Input: dimensioned drawing with shaded views. Units: mm. Origin: part minimum x, y, z. A direction names the side the tool comes from. Give positions to 0.01 mm unless a question says otherwise; leave off trailing zeros. Write each loop counter-clockwise with the first axis right and the second up, starting at its lowest first coordinate (ties: lowest second). Pieces come first, ordered by that corner, then holes. Notation, with made-up numbers: M 10.5,44 L 46.5,44 A28 cw 46.5,69 Z; hole C 24,78 d7. An arc over 180 degrees is marked long. Answer as a JSON object with one key per item and string values.
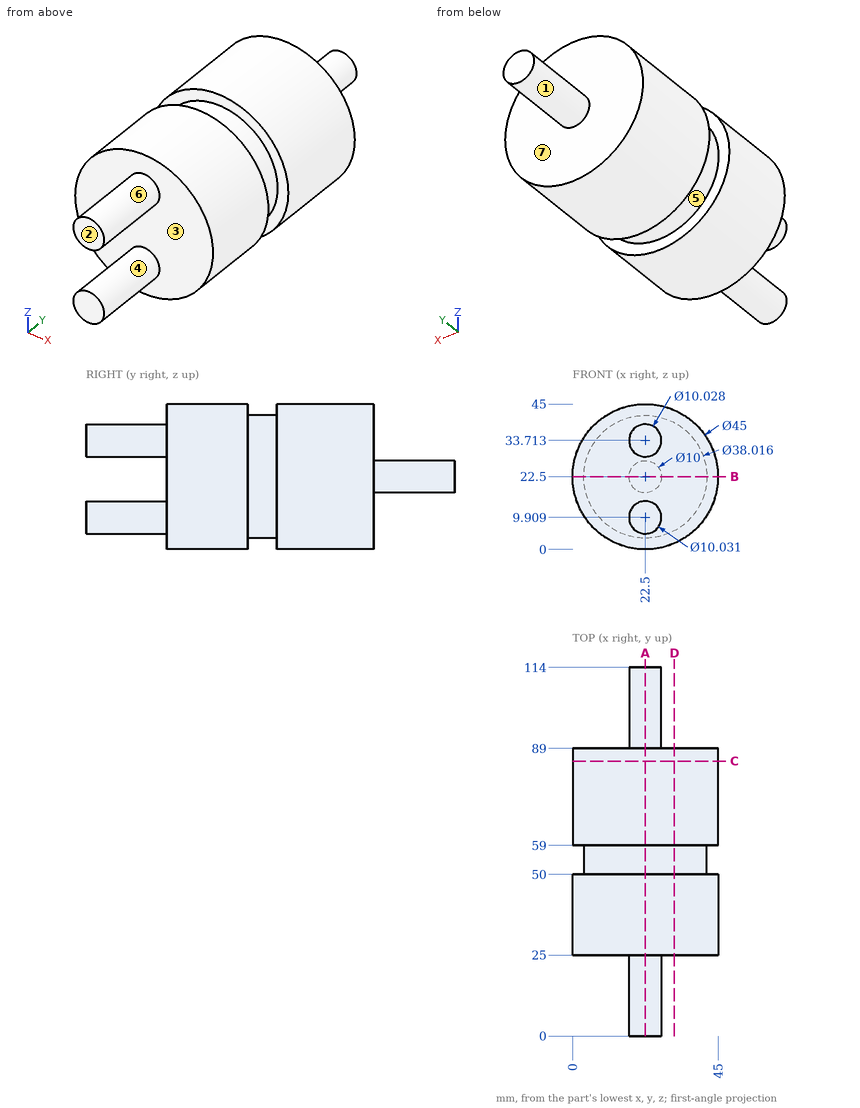
1) Cut plane A-A on x = 22.5. Return loops of the section in (y, z) (1 decimal), and give its area (3 significant figures).
Geometry check:
{"outline": "M 0,4.9 L 25,4.9 L 25,0 L 50,0 L 50,3.5 L 59,3.5 L 59,0 L 89,0 L 89,17.5 L 114,17.5 L 114,27.5 L 89,27.5 L 89,45 L 59,45 L 59,41.5 L 50,41.5 L 50,45 L 25,45 L 25,38.7 L 0,38.7 L 0,28.7 L 25,28.7 L 25,14.9 L 0,14.9 Z", "area": "3,570 mm2"}
2) Contact query for flat-ended pins moving along their axis: P1, Ø3, axis at x = 24.5, y = 67, coming from the +Z side; P2, Ø2, axis at y = 81, z = 29, coming from the -X side; P3, Ø22.5, axis at x = 17, z = 19.5, coming from the +Y side; P4, Ø5, axis at x = 39, z = 5, coming from the -Y side. Output: stop coordinate, or through.
Geometry check:
{"P1": "stops at z = 44.99", "P2": "stops at x = 0.68", "P3": "stops at y = 114", "P4": "stops at y = 25"}
3) Set-up query: the marked faces 1, 2 and 3. Return all of +Z, -Z, +X, -X, +Y, -Y with unobstructed straight access to the full face (end or side cutting, diameter ignored); none if empty.
Geometry check:
{"face 1": "+Y", "face 2": "+Z, -Z, +X, -X, -Y", "face 3": "-Y"}
4) Cut plane D-D on x = 31.5. Return loops of the section in (y, z), and give its area (3 significant figures).
Geometry check:
{"outline": "M 25,1.88 L 50,1.88 L 50,5.76 L 59,5.76 L 59,1.88 L 89,1.88 L 89,43.12 L 59,43.12 L 59,39.24 L 50,39.24 L 50,43.12 L 25,43.12 Z", "area": "2,570 mm2"}
5) Cut plane B-B on z = 22.5. Return loops of the section in (x, y), and give its area (3 significant figures).
Geometry check:
{"outline": "M 0,25 L 45,25 L 45,50 L 41.51,50 L 41.51,59 L 45,59 L 45,89 L 27.5,89 L 27.5,114 L 17.5,114 L 17.5,89 L 0,89 L 0,59 L 3.49,59 L 3.49,50 L 0,50 Z", "area": "3,070 mm2"}
6) Line query: line 1 (Y direction, x = 4.5, z = 9.5); line 2 (Y direction, x = 19, z = 17.5); line 3 (X direction, y = 26, z = 22) (1 decimal). Output: solid intervals per line, ascending. Write a range as from..to.
Geometry check:
{"line 1": "y = 25..50, 59..89", "line 2": "y = 25..89", "line 3": "x = 0..45"}
7) Cut plane C-C on y = 85. Return loops of the section in (x, z), and give its area (3 significant figures).
Geometry check:
{"outline": "C 22.5,22.5 d45", "area": "1,590 mm2"}
8) Pull-direction query (Z, two-part tool) for the marked faces 4, 5, 6 and 7; classes: pulls with the +Z half, pulls with the -Z half, needs draft (parallel to the pull), parting line crosses it, or undercut.
Geometry check:
{"face 4": "undercut", "face 5": "parting line crosses it", "face 6": "undercut", "face 7": "needs draft"}
